Autodesk Fusion 360 part; units mm, degrees
sketch "Sketch1" plane through (0, 0, 0) normal (0, 1, 0) x (1, 0, 0)
  line L0 (0, 0) -> (8, 0)
  line L1 (8, 0) -> (8, 10)
  line L2 (8, 10) -> (0, 10)
  line L3 (0, 10) -> (0, 0)
  dimension "d1" = 8
  dimension "d2" = 10
extrude "Extrude1" add sketch "Sketch1" along normal blind 2
sketch "Sketch3" plane through (0, 2, 0) normal (0, 1, 0) x (-1, 0, 0)
  line L0 (0, -10) -> (0, 0)
  line L1 (0, 0) -> (-8, 0)
  line L2 (-8, 0) -> (-8, -10)
  line L3 (-8, -10) -> (0, -10)
  line L4 (0, 0) -> (-2, 0)
  line L5 (-2, 0) -> (-2, -10)
  line L6 (-2, -10) -> (0, -10)
  line L7 (0, -10) -> (0, 0)
  line L8 (-8, 0) -> (-6, 0)
  line L9 (-6, 0) -> (-6, -10)
  line L10 (-6, -10) -> (-8, -10)
  line L11 (-8, -10) -> (-8, 0)
  dimension "d5" = 2
  dimension "d6" = 2
extrude "Extrude2" add sketch "Sketch3" along normal blind 3 contours L0 L1 L3 L4 L5 L6 L7 | L1 L2 L3 L8 L9 L10 L11
Build history of the part. All positions in model axes, mm. A direction names the side the tool comes from. Round coordinates to 2 decimals unless told otherwise and drop trailing zeros. Loops run counter-clockwise (first coordinate to the right, second up) from the corner with the lowest first, then second, coordinate; pieces in that order, holes last.
Item 1: Pin check, flat tip, straight feed: P1, Ø1, axis at x = 5.5, z = -5.5, coming from the -Y side. Stop position of the tip, or through.
Item 2: Which spindle directions (+Z, -Z, +X, -X, +Y, -Y) get a long thin tool onto all of the face, cutting with end or side? Do faces 4 (the face through (6, 3, -5)), 5 (the face through (8, 2, -5)). Say none if no direction does.
Item 3: Saw through at B-B (z = -3.75). List the corners of the cut face in (x, y), then the cut area to 3 significant figures.
Item 4: Drill centre lines: line 1 along X through (y, z) = (2.6, -3.25); line 2 along Y through (x, z) = (3, -7.75). Where is each one in solid material? Low to high.
Item 5: Saw through at A-A (y = 4.15). List the corners of the cut face in (x, z), then the cut area to 3 significant figures.
Item 6: Two-plate mould, pull along X, no slides. Class faces 1 (the face through (4, 0, -5)), 2 (the face through (2, 3, -5)), 3 (the face through (0, 2, -5)): released by +X, released by -X, zero draft, split by the parting line, or undercut.
Item 7: Saw through at C-C (x = 4.25). List the corners of the cut face in (y, z), then the cut area to 3 significant figures.
Worked answers:
1. P1: stops at y = 0
2. face 4: +Z, -Z, +Y
2. face 5: +Z, -Z, +X, +Y, -Y
3. outline: (0, 0) - (8, 0) - (8, 5) - (6, 5) - (6, 2) - (2, 2) - (2, 5) - (0, 5) - close
3. area: 28.0 mm2
4. line 1: x = 0 to 2, 6 to 8
4. line 2: y = 0 to 2
5. outline: (0, -10) - (2, -10) - (2, 0) - (0, 0) - close; (6, -10) - (8, -10) - (8, 0) - (6, 0) - close
5. area: 40.0 mm2
6. face 1: zero draft
6. face 2: undercut
6. face 3: released by -X
7. outline: (0, -10) - (2, -10) - (2, 0) - (0, 0) - close
7. area: 20.0 mm2
